Verification items for the finished model (mm, model axes). A direction names the side the tool comes from. Round coordinates to 2 decimals unless told otherwise and drop trailing zeros. Loops run counter-clockwise (first coordinate to the right, second up) from the corner with the lowest first, then second, coordinate; pieces in that order, holes last.
Autodesk Inventor part; units mm, degrees
ref_plane "Plano inicial" through (0, 0, 25) normal (0, 0, 1) x (1, 0, 0)
ref_plane "Plano final" through (0, 0, 380) normal (0, 0, 1) x (1, 0, 0)
ref_plane "Plano de trabajo4" through (-350.06, 21, 380) normal (0, 0, 1) x (1, 0, 0)
ref_plane "Plano inicial" through (0, 0, 25) normal (0, 0, 1) x (1, 0, 0)
ref_plane "Plano final" through (0, 0, 380) normal (0, 0, 1) x (1, 0, 0)
sketch "Boceto" plane through (0, 0, 0) normal (0, 0, 1) x (1, 0, 0)
  line L0 (-25, -21) -> (-25, 21)
  line L1 (-21, 25) -> (21, 25)
  line L2 (25, 21) -> (25, -21)
  line L3 (21, -25) -> (-21, -25)
  arc A0 (-25, -21) -> (-21, -25) centre (-21, -21) ccw
  arc A1 (25, 21) -> (21, 25) centre (21, 21) ccw
  arc A2 (-21, 25) -> (-25, 21) centre (-21, 21) ccw
  arc A3 (21, -25) -> (25, -21) centre (21, -21) ccw
  arc A4 (-21, 23) -> (-23, 21) centre (-21, 21) ccw
  line L4 (-21, 23) -> (21, 23)
  arc A5 (23, 21) -> (21, 23) centre (21, 21) ccw
  line L5 (23, 21) -> (23, -21)
  arc A6 (21, -23) -> (23, -21) centre (21, -21) ccw
  line L6 (21, -23) -> (-21, -23)
  arc A7 (-23, -21) -> (-21, -23) centre (-21, -21) ccw
  line L7 (-23, -21) -> (-23, 21)
  line L8 (0, 36.1598) -> (0, -36.1598) construction
  line L9 (-36.1598, 0) -> (36.1598, 0) construction
  dimension "d7" = 4
  dimension "d9" = 50
  dimension "d11" = 50
  dimension "d12" = 2
  dimension "d15" = 25
  dimension "d16" = 25
extrude "Cuerpo" add sketch "Boceto" along normal up to surface (355 mm away) from surface at 25
sketch "Sketch3" plane through (0, 0, 0) normal (0, 0, 1) x (1, 0, 0)
  line L0 (0, 0) -> (10, 0)
ref_plane "Work Plane3" through (0, 0, 0) normal (0, -1, 0) x (1, 0, 0)
sketch "Sketch4" plane through (0, 0, 0) normal (0, -1, 0) x (1, 0, 0)
  line L0 (-2, 25) -> (12, 25)
  line L1 (-2, 380) -> (12, 380)
  dimension "d18" = 355
ref_plane "Plano de trabajo4" through (-350.06, 21, 380) normal (0, 0, 1) x (1, 0, 0)
split "Dividir1" plane through (-350.06, 21, 380) removes the side toward (0, 0, 1)
ref_plane "Plano de trabajo5" through (-350.06, -21, 25) normal (0, 0, -1) x (-1, 0, 0)
split "Dividir2" plane through (-350.06, -21, 25) removes the side toward (0, 0, -1)
equation "\"d7\" = G_IR"
equation "\"d9\" = G_W"
equation "\"d11\" = G_H"
equation "\"d12\" = G_T"
equation "\"d15\" = 0.5 * d9"
equation "\"d16\" = 0.5 * d11"
equation "\"d3\" = G_L"
equation "\"G_W\" = 50"
equation "\"G_H\" = 50"
equation "\"G_T\" = 2"
equation "\"G_IR\" = 4"
equation "\"G_L\" = d18"
equation "\"G_OFFSET_START\" = -25"
equation "\"G_OFFSET_END\" = -25"
equation "\"d13\" = -G_OFFSET_START"
equation "\"B_L\" = 405"
properties part number "ISO 10799-2 - 50x50x2 - 355" material "Galvanizado catalogo 1"
1. Tool access check on faces 1 (the face through (0, 24, 25)), 2 (the face through (0, -23, 200)). Record the directions out of +Z, -Z, +X, -X, +Y, -Y that give a thin tool (end or side, any length) a straight path to the whole face; none if there is none.
2. Scan lines: L1, parallel to X at y = 2.5, z = 70.5; L2, parallel to X at y = -21.5, z = 338. Record each from-to range of solid material in increasing order.
3. Section check B-B (y = 1.5). Enter the section's corners in (x, z).
4. Section check A-A (z = 185). Enter the section's corners in (x, y), then the cut area to 3 significant figures.
5. Release check for a two-part mould opening along X. For faces 3 (the face through (-25, 0, 200)), 4 (the face through (0, -25, 200)), 5 (the face through (23, 0, 200)), 6 (the face through (-23, 0, 200)) record: released by +X, released by -X, zero draft, split by the parting line, or undercut.
Taken from the geometry:
1. face 1: -Z, +X, -X, +Y, -Y
1. face 2: +Z, -Z
2. L1: x = -25 to -23, 23 to 25
2. L2: x = -24.97 to -22.94, 22.94 to 24.97
3. outline: (-25, 25) - (-23, 25) - (-23, 380) - (-25, 380) - close; (23, 25) - (25, 25) - (25, 380) - (23, 380) - close
4. outline: (-25, -21) arc R4 ccw to (-21, -25) - (21, -25) arc R4 ccw to (25, -21) - (25, 21) arc R4 ccw to (21, 25) - (-21, 25) arc R4 ccw to (-25, 21) - close; hole (-23, -21) arc R2 ccw to (-21, -23) - (21, -23) arc R2 ccw to (23, -21) - (23, 21) arc R2 ccw to (21, 23) - (-21, 23) arc R2 ccw to (-23, 21) - close
4. area: 374 mm2
5. face 3: released by -X
5. face 4: zero draft
5. face 5: undercut
5. face 6: undercut
